from build123d import *

# Parameters (mm, degrees)
SKETCH2_R               = 6.35
BOSS_EXTRUDE1_DEPTH     = 25.4
SKETCH3_R               = 3.175
CUT_EXTRUDE1_DEPTH      = 7.35
CUT_EXTRUDE1_DEPTH_BACK = 7.35


with BuildPart() as part:
    # Sketch2 → Boss-Extrude1 (new body)
    with BuildSketch(Plane.XY):
        Circle(SKETCH2_R)
    extrude(amount=BOSS_EXTRUDE1_DEPTH)

    # Sketch3 → Cut-Extrude1 (cut, two sides)
    with BuildSketch(Plane(origin=(0, 0, 0), x_dir=(1, 0, 0), z_dir=(0, 1, 0))) as cut_extrude1_sk:
        with Locations(Location((0, -12.7, 0), (0, 0, 270))):  # turned: the seam where the file's is
            Circle(SKETCH3_R)
    extrude(amount=CUT_EXTRUDE1_DEPTH, mode=Mode.SUBTRACT)
    extrude(cut_extrude1_sk.sketch, amount=-CUT_EXTRUDE1_DEPTH_BACK, mode=Mode.SUBTRACT)

    # Sketch7 → Revolve2 (revolve)
    with BuildSketch(Plane(origin=(0, 0, 0), x_dir=(1, 0, 0), z_dir=(0, 1, 0))):
        with BuildLine():
            Line((-69.85, 6.35), (-76.2, 6.35))
            Line((-76.2, 6.35), (-76.2, 0))
            Line((-76.2, 0), (0, 0))
            Line((0, 0), (0, 3.175))
            ThreePointArc((0, 3.175), (-34.961060929, 3.969159572), (-69.85, 6.35))
        make_face()
    revolve(axis=Axis((0, 0, 50), (0, 0, -1)))


solid = part.part
Verification items for the finished model (mm, model axes). A direction names the side the tool comes from. Coordinates: 2 decimals unless noted, no trailing zeros. Write each loop counter-clockwise with the first axis right and the second up, starting at its lowest first coordinate (ties: lowest second). Pieces come first, ordered by that corner, then holes. Notation, with made-up numbers: M 28.5,82 L 59.5,82 A24 ccw 59.5,107 Z; hole C -13,-24 d6. An arc over 180 degrees is marked long. Use CSV: the item, a comma, the result in double quotes.
Q1. Section check C-C, the plane x = -61.5. Enter the section's corners in (y, z), and give its area (3 significant figures).
Computed values:
outline,"M -44.99,-6.35 L -33.12,-6.35 A767.48 cw 33.12,-6.35 L 44.99,-6.35 L 44.99,0 L -44.99,0 Z"
area,"540 mm²"
Q2. Section check B-B, the plane z = 21. Enter the section's corners in (x, y), and give its area (3 significant figures).
Computed values:
outline,"C 0,0 d12.7"
area,"127 mm²"
Q3. Set-up check for faces 1 (the flat face through (0, 0, 25.4)), 2 (the cylindrical face through (5.866, -2.432, 12.522)): record each of +Z, -Z, +X, -X, +Y, -Y from which the full face is reachable in a straight line by a thin tool's end or side.
Computed values:
face 1,"+Z, +X, -X, +Y, -Y"
face 2,"+Z"
Q4. Go/stop test with flat-tipped pins: P1, Ø5, axis at x = -39.5, z = 3, coming from the -Y side; P2, Ø12, axis at x = -20.5, y = -59.5, coming from the +Z side; P3, Ø8, axis at x = 19.5, y = 12, coming from the -Z side; P4, Ø3, axis at x = -53, y = -23.5, coming from the -Z side. Record where each tip stops, or that it passes through.
Computed values:
P1,"through"
P2,"z = 0"
P3,"z = -3.64"
P4,"z = -5.48"
Q5. Thickness scan on line 1 along Z through (x, y) = (0, -1.75) (3 decimals); line 2 along X through (y, z) = (-45, -0.5); line 3 along Y through (x, z) = (-27.5, -1). Record the ranges inside material, lowest first. Write a range as [from, to].
Computed values:
line 1,"[-3.177, 9.525], [15.875, 25.4]"
line 2,"[-61.49, 61.49]"
line 3,"[-71.06, 71.06]"
Q6. Section check D-D, the plane y = -11.5. Enter the section's corners in (x, z), and give its area (3 significant figures).
Computed values:
outline,"M -75.33,-6.35 L -68.9,-6.35 A769.85 cw 68.9,-6.35 L 75.33,-6.35 L 75.33,0 L -75.33,0 Z"
area,"673 mm²"
